Design review of the part built by this model. Coordinates are the model's own, in mm. Round coordinates to 2 decimals unless told otherwise and drop trailing zeros. Order: outer loops, then holes, each group sorted by start corner. A loop starts at its lowest first (then second) coordinate and runs counter-clockwise, first axis right, second up. Notation, with made-up numbers: (85.5, 86) - (109.5, 86) arc R24 cw to (109.5, 105) - close; hole circle Ø6 at (20.25, -4). An arc over 180 degrees is marked (long way). Use CSV: the item, a comma, the result in double quotes. Start each with the question number.
from build123d import *

# Parameters (mm, degrees)
SKETCH_1_R      = 3
EXTRUDE_1_DEPTH = 3
FILLET_1_R      = 1


with BuildPart() as part:
    # 草图1 → 凸台-拉伸1 (new body)
    with BuildSketch(Plane(origin=(0, 0, 0), x_dir=(0, 0, -1), z_dir=(1, 0, 0))):
        with BuildLine():
            Line((-34, 7), (34, 7))
            ThreePointArc((34, 7), (41, 0), (34, -7))
            Line((34, -7), (-34, -7))
            ThreePointArc((-34, -7), (-41, 0), (-34, 7))
        make_face()
        with Locations((-34, 0)):
            Circle(SKETCH_1_R, mode=Mode.SUBTRACT)
        with Locations((34, 0)):
            Circle(SKETCH_1_R, mode=Mode.SUBTRACT)
    extrude(amount=EXTRUDE_1_DEPTH)

    # 圆角1
    fillet_1_edges = [part.edges().sort_by_distance(p)[0] for p in [
        (3, 0, -41),
        (3, 7, 0),
        (3, 0, 41),
        (0, 7, 0),
        (0, 0, -41),
        (0, -7, 0),
        (0, 0, 41),
        (3, -7, 0),
    ]]
    fillet(fillet_1_edges, radius=FILLET_1_R)


solid = part.part
Q1. Take a section at C-C (z = 2). State the section outline as (x, y) points, plus the area to 3 significant figures.
Q2. Take a section at A-A (y = 0). State the section outline as (x, z) points, plus the area to 3 significant figures.
Q3. The part is to be moulded in two halves that separate along Z. For faces 1 (the flat face through (0, 0, -1)), 2 (the cylindrical face through (1, 0, 37)), 3 (the cylindrical face through (1.49, -0.15, 41)), 4 (the cylindrical face through (1, 0, -31)), say which applies: +Z half, -Z half, draft (parallel to the pull), parting line (faces both ways), or undercut.
Q4. For L1, parallel to Z at x = 1.55, y = 1.75; L2, parallel to Z at x = 0.6, y = 2; L3, parallel to Y at x = 2.4, z = 35, list the stretches that pass through material, from the lowest coordinate up. Write a range as [from, to].
Q5. Take a section at B-B (z = -32). State the section outline as (x, y) points.
Q6. Clearance check with a flat-ended pin moving along its axis: pin 1 (1 mm diameter, centred on x = 2.5, y = 1.5, fed in from -Z). State where the tip first meets the part, or that it passes through.
Findings below:
1,outline,"(0, -6) arc R1 ccw to (1, -7) - (2, -7) arc R1 ccw to (3, -6) - (3, 6) arc R1 ccw to (2, 7) - (1, 7) arc R1 ccw to (0, 6) - close"
1,area,"41.1 mm^2"
2,outline,"(0, -40) arc R1 ccw to (1, -41) - (2, -41) arc R1 ccw to (3, -40) - (3, -37) - (0, -37) - close; (0, -31) - (3, -31) - (3, 31) - (0, 31) - close; (0, 37) - (3, 37) - (3, 40) arc R1 ccw to (2, 41) - (1, 41) arc R1 ccw to (0, 40) - close"
2,area,"209 mm^2"
3,face 1,"draft"
3,face 2,"undercut"
3,face 3,"+Z half"
3,face 4,"undercut"
4,L1,"z = [-40.78, -36.44], [-31.56, 31.56], [36.44, 40.78]"
4,L2,"z = [-40.62, -36.24], [-31.76, 31.76], [36.24, 40.62]"
4,L3,"y = [-6.84, -2.83], [2.83, 6.84]"
5,outline,"(0, -6) arc R1 ccw to (1, -7) - (2, -7) arc R1 ccw to (3, -6) - (3, -2.24) - (0, -2.24) - close; (0, 2.24) - (3, 2.24) - (3, 6) arc R1 ccw to (2, 7) - (1, 7) arc R1 ccw to (0, 6) - close"
6,pin 1,"stops at z = -40.89"
